Source: CAD feature listing. Evaluate the final solid. Frame: model axes, mm. Face numbers are marked on the shaded views. Give positions to 0.01 mm unless a question says otherwise; leave off trailing zeros. Loops run counter-clockwise (first coordinate to the right, second up) from the corner with the lowest first, then second, coordinate; pieces in that order, holes last. Notation, with made-up numbers: (76, -19.75) -> (116, -19.75) arc R16 ccw to (116, -8.75) -> close; hole circle Ø6 at (-14, 67). An arc over 180 degrees is marked (long way). Return JSON: item names as keys, results as strings. Group by question number.
(1) Pin query (flat end, axial travel): pin 1 (11 mm diameter, centred on y = -30.84, z = 52.45, fed in from +X); pin 2 (17.5 mm diameter, centred on y = 60, z = 0, fed in from -X); pin 3 (3 mm diameter, centred on x = 9, y = -12, fed in from +Z); pin 4 (6 mm diameter, centred on x = 3, y = -17.5, fed in from +Z). Return the tip coordinate at first contact, or that it passes through.
(2) Ray query, line 1 (Y direction, x = 3.25, z = 0); line 2 (Z direction, x = 7.25, y = 34); line 3 (Y direction, x = 5, z = -56). Return the intervals inside material, ascending. Write a range as from..to.
(3) Cut plane B-B on z = 0. Return loops of the section in (x, y).
(4) Draft query along Y for the marked faces 1, 2 and 3. Return one class per face: released by +Y, released by -Y, zero draft, split by the parting line, or undercut.
(5) Cut plane C-C on x = 7. Return loops of the section in (y, z), then the cut area to 3 significant figures.
(6) Cut plane D-D on z = 24. Return loops of the section in (x, y).
(7) Cut plane A-A on y = 0. Return loops of the section in (x, z), then the cut area to 3 significant figures.
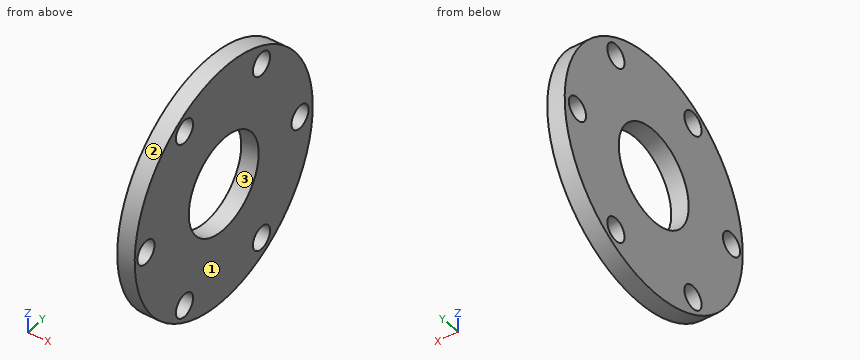
```python
from build123d import *

# Parameters (mm, degrees)
CROQUIS1_R              = 70
SALIENTE_EXTRUIR1_DEPTH = 10
MATRIZC5_COUNT          = 6
CROQUIS9_R              = 27.5
CORTAR_EXTRUIR1_DEPTH   = 10


with BuildPart() as part:
    # Croquis1 → Saliente-Extruir1 (new body)
    with BuildSketch(Plane(origin=(0, 0, 0), x_dir=(0, 0, -1), z_dir=(1, 0, 0))):
        Circle(CROQUIS1_R)
    extrude(amount=SALIENTE_EXTRUIR1_DEPTH)

    # Croquis8 → Taladro de margen para M122 (revolve, cut)
    with BuildSketch(Plane(origin=(10, 60, 0), x_dir=(0, 0, -1), z_dir=(0, 1, 0))):
        Polygon((0, 0), (0, 47.555809178), (6.75, 43.5), (6.75, 0), align=None)
    taladro_de_margen_para_m122 = revolve(axis=Axis((16.35, 60, 0), (-1, 0, 0)), mode=Mode.SUBTRACT)

    # MatrizC5: Taladro de margen para M122 ×6 about axis
    matrizc5_axis = Axis((0, -0.563144546, 0), (1, 0, 0))
    for i in range(1, MATRIZC5_COUNT):
        add(taladro_de_margen_para_m122.rotate(matrizc5_axis, i * 360 / MATRIZC5_COUNT), mode=Mode.SUBTRACT)

    # Croquis9 → Cortar-Extruir1 (cut)
    with BuildSketch(Plane(origin=(10, 0, 0), x_dir=(0, 0, -1), z_dir=(1, 0, 0))):
        Circle(CROQUIS9_R)
    extrude(amount=-CORTAR_EXTRUIR1_DEPTH, mode=Mode.SUBTRACT)


solid = part.part
```
Answers:
{
 "1": {"pin 1": "through", "pin 2": "x = 0", "pin 3": "z = 69.21", "pin 4": "z = 68.48"},
 "2": {"line 1": "-70..-67.88, -54.38..-27.5, 27.5..53.25, 66.75..70", "line 2": "-61.19..-57.67, -47.23..47.23, 57.67..61.19", "line 3": "-42..-36.59, -25.1..23.98, 35.46..42"},
 "3": {"outline": "(0, -70) -> (10, -70) -> (10, -67.88) -> (0, -67.88) -> close; (0, -54.38) -> (10, -54.38) -> (10, -27.5) -> (0, -27.5) -> close; (0, 27.5) -> (10, 27.5) -> (10, 53.25) -> (0, 53.25) -> close; (0, 66.75) -> (10, 66.75) -> (10, 70) -> (0, 70) -> close"},
 "4": {"face 1": "zero draft", "face 2": "split by the parting line", "face 3": "undercut"},
 "5": {"outline": "circle Ø140 at (0, 0); hole circle Ø13.5 at (-61.13, 0); hole circle Ø13.5 at (-30.84, -52.45); hole circle Ø13.5 at (-30.84, 52.45); hole circle Ø55 at (0, 0); hole circle Ø13.5 at (29.72, -52.45); hole circle Ø13.5 at (29.72, 52.45); hole circle Ø13.5 at (60, 0)", "area": "12,200 mm²"},
 "6": {"outline": "(0, -65.76) -> (10, -65.76) -> (10, -13.43) -> (0, -13.43) -> close; (0, 13.43) -> (10, 13.43) -> (10, 65.76) -> (0, 65.76) -> close"},
 "7": {"outline": "(0, -70) -> (10, -70) -> (10, -27.5) -> (0, -27.5) -> close; (0, 27.5) -> (10, 27.5) -> (10, 70) -> (0, 70) -> close", "area": "850 mm²"}
}
